from build123d import *

# Parameters (mm, degrees)
F0_W     = 31.75
F0_H     = 31.75
F0_W_2   = 6.35
F0_H_2   = 6.35
F0_R     = 1.5875
F1_DEPTH = 7.9375
F2_DEPTH = 3.175


# Not quite as in the source:
# - a length typed as a fraction of an inch, garbled in the dataset ("3 / 203.2 mm" for 3/8 in), is restored


with BuildPart() as f1:
    # F0 (on Front) → F1 (new body)
    with BuildSketch(Plane.XZ):
        Rectangle(F0_W, F0_H)
        with Locations((-6.35, -6.35)):
            Rectangle(F0_W_2, F0_H_2, mode=Mode.SUBTRACT)
        with Locations((0, -6.35)):
            Circle(F0_R, mode=Mode.SUBTRACT)
        with Locations((6.35, -6.35)):
            Rectangle(F0_W_2, F0_H_2, mode=Mode.SUBTRACT)
        with Locations((-6.35, 0)):
            Circle(F0_R, mode=Mode.SUBTRACT)
        with Locations((-6.35, 6.35)):
            Rectangle(F0_W_2, F0_H_2, mode=Mode.SUBTRACT)
        Circle(F0_R, mode=Mode.SUBTRACT)
        with Locations((6.35, 0)):
            Circle(F0_R, mode=Mode.SUBTRACT)
        with Locations((0, 6.35)):
            Circle(F0_R, mode=Mode.SUBTRACT)
        with Locations((6.35, 6.35)):
            Circle(F0_R, mode=Mode.SUBTRACT)
    extrude(amount=F1_DEPTH)

    # F0 (on Front) → F2 (join)
    with BuildSketch(Plane.XZ):
        Rectangle(F0_W, F0_H)
        with Locations((-6.35, -6.35)):
            Rectangle(F0_W_2, F0_H_2, mode=Mode.SUBTRACT)
        with Locations((0, -6.35)):
            Circle(F0_R, mode=Mode.SUBTRACT)
        with Locations((6.35, -6.35)):
            Rectangle(F0_W_2, F0_H_2, mode=Mode.SUBTRACT)
        with Locations((-6.35, 0)):
            Circle(F0_R, mode=Mode.SUBTRACT)
        with Locations((-6.35, 6.35)):
            Rectangle(F0_W_2, F0_H_2, mode=Mode.SUBTRACT)
        Circle(F0_R, mode=Mode.SUBTRACT)
        with Locations((6.35, 0)):
            Circle(F0_R, mode=Mode.SUBTRACT)
        with Locations((0, 6.35)):
            Circle(F0_R, mode=Mode.SUBTRACT)
        with Locations((6.35, 6.35)):
            Circle(F0_R, mode=Mode.SUBTRACT)
        with Locations((6.35, -6.35)):
            Rectangle(F0_W_2, F0_H_2)
        with Locations((-6.35, -6.35)):
            Rectangle(F0_W_2, F0_H_2)
        with Locations((-6.35, 6.35)):
            Rectangle(F0_W_2, F0_H_2)
        with Locations((-6.35, 0)):
            Circle(F0_R)
        Circle(F0_R)
        with Locations((0, -6.35)):
            Circle(F0_R)
        with Locations((6.35, 0)):
            Circle(F0_R)
        with Locations((6.35, 6.35)):
            Circle(F0_R)
        with Locations((0, 6.35)):
            Circle(F0_R)
    extrude(amount=F2_DEPTH)


solid = f1.part
Geometry: final body of the model. Coordinates: model frame, mm. Give positions to 0.01 mm unless a question says otherwise; leave off trailing zeros. Write each loop counter-clockwise with the first axis right and the second up, starting at its lowest first coordinate (ties: lowest second). Pieces come first, ordered by that corner, then holes. Notation, with made-up numbers: M 17.25,-23.5 L 49.25,-23.5 A18 cw 49.25,10.5 Z; hole C -25,19.5 d11. An arc over 180 degrees is marked long. Answer in a Markdown table with one row per item. Add a question column.
(1) Section B-B on x = 0. Return loops of the section in (y, z) (1 decimal), and give its area (3 significant figures).
(2) Section C-C on z = -6.35. Return loops of the section in (x, y) (1 decimal).
(3) Section A-A on y = -6.25. State how many separate pieces and enclosed holes the cut face has, and give its area (3 significant figures).
(4) Ray query, line 1 (X direction, y = -4.25, z = 6.35) (1 decimal); line 2 (Z direction, x = 0, y = -4.45) (1 decimal); line 3 (X direction, y = -4.5, z = -6.35) (1 decimal). Return the intervals inside material, ascending.
(5) Mould query, pull axis Z, two halves, no side actions, for faces 1 (the flat face through (0, -4, 15.875)), 2 (the cylindrical face through (0.73, -5.52, 4.94)). Classes: +Z half, -Z half, draft (parallel to the pull), parting line (faces both ways), or undercut.
(6) First-contact query: pin 1 (1 mm diameter, centred on x = -6.5, z = 4, fed in from +Y); pin 2 (1.9 mm diameter, centred on x = -6, z = -5, fed in from -Y) (3 decimals). Flat tips, straight axial feed; report the tip coordinate or a pass-through.
Result set:
| question | item | result |
|---|---|---|
| 1 | outline | M -7.9,-15.9 L 0,-15.9 L 0,15.9 L -7.9,15.9 L -7.9,7.9 L -3.2,7.9 L -3.2,4.8 L -7.9,4.8 L -7.9,1.6 L -3.2,1.6 L -3.2,-1.6 L -7.9,-1.6 L -7.9,-4.8 L -3.2,-4.8 L -3.2,-7.9 L -7.9,-7.9 Z |
| 1 | area | 207 mm^2 |
| 2 | outline | M -15.9,-7.9 L -9.5,-7.9 L -9.5,-3.2 L -3.2,-3.2 L -3.2,-7.9 L -1.6,-7.9 L -1.6,-3.2 L 1.6,-3.2 L 1.6,-7.9 L 3.2,-7.9 L 3.2,-3.2 L 9.5,-3.2 L 9.5,-7.9 L 15.9,-7.9 L 15.9,0 L -15.9,0 Z |
| 3 | separate pieces | 1 |
| 3 | enclosed holes | 9 |
| 3 | area | 840 mm^2 |
| 4 | line 1 | x = -15.9 to -9.5, -3.2 to -1.6, 1.6 to 4.8, 7.9 to 15.9 |
| 4 | line 2 | z = -15.9 to -7.9, -4.8 to -1.6, 1.6 to 4.8, 7.9 to 15.9 |
| 4 | line 3 | x = -15.9 to -9.5, -3.2 to -1.6, 1.6 to 3.2, 9.5 to 15.9 |
| 5 | face 1 | +Z half |
| 5 | face 2 | undercut |
| 6 | pin 1 | stops at y = 0 |
| 6 | pin 2 | stops at y = -3.175 |
